Study the drawing (mm; zero at the part's minimum x, y, z) and answer. A direction names the side the tool comes from. Give positions to 0.01 mm unless a question says otherwise; leave off trailing zeros. Order: outer loops, then holes, each group sorted by start corner. A loop starts at its lowest first (then second) coordinate and runs counter-clockwise, first axis right, second up. Notation, with made-up numbers: (-2, 70.25) - (38, 70.25) arc R13 ccw to (38, 88.25) - close; hole circle Ø2 at (49.25, 86). An arc over 180 degrees is marked (long way). Put each result on its own line as item: value.
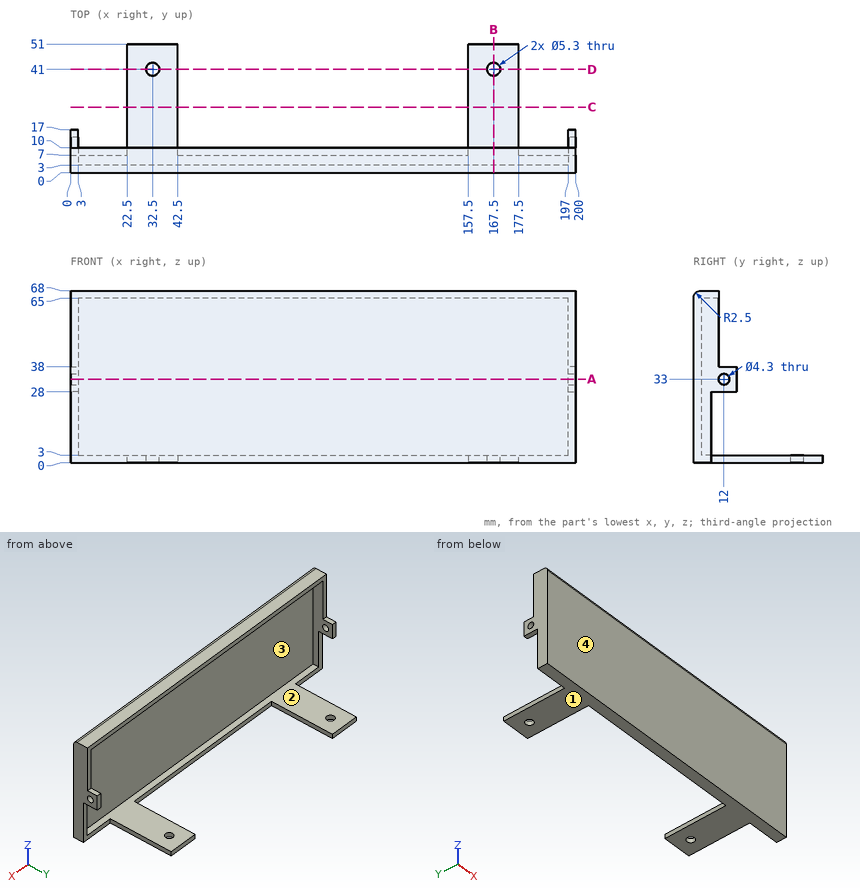
(1) Given pin 1 (18 mm diameter, centred on x = 193, z = 12, fed in from +Y); pin 2 (2.5 mm diameter, centred on y = 19, z = 1.5, fed in from +X); pin 3 (0.9 mm diameter, centred on x = 1, y = 13.5, fed in from -Z); pin 4 (2.5 mm diameter, centred on y = 12, z = 33, fed in from +X), each flat-ended and moving along its own axis, determine where each tip first touches the part or whether it passes through.
Geometry check:
pin 1: stops at y = 7
pin 2: stops at x = 177.5
pin 3: stops at z = 28
pin 4: passes through
(2) Section A-A, the plane z = 33 is taken. Write down the section's boundary in (x, y).
Geometry check:
outline: (0, 0) - (200, 0) - (200, 9.85) - (197, 9.85) - (197, 3) - (3, 3) - (3, 9.85) - (0, 9.85) - close; (0, 14.15) - (3, 14.15) - (3, 17) - (0, 17) - close; (197, 14.15) - (200, 14.15) - (200, 17) - (197, 17) - close
(3) A tool of negligible diameter and unlimited length cuts with its end or side. For the marked faces 3 and 4, from which of +Z, -Z, +X, -X, +Y, -Y can it reach the whole face along a straight path? Write none if from no direction.
Geometry check:
face 3: +Y
face 4: +Z, -Z, +X, -X, -Y
(4) Determine the mould class of the marked faces 1 and 2 for opening direction X: pulls with the +X half, pulls with the -X half, needs draft (parallel to the pull), parting line crosses it, or undercut.
Geometry check:
face 1: needs draft
face 2: undercut
(5) Section C-C, the plane y = 26 is taken. Write down the section's boundary in (x, z).
Geometry check:
outline: (22.5, 0) - (42.5, 0) - (42.5, 3) - (22.5, 3) - close; (157.5, 0) - (177.5, 0) - (177.5, 3) - (157.5, 3) - close
(6) Straight lines are drawn through the part: line 1 (X direction, y = 41, z = 1); line 2 (X direction, y = 9, z = 51); line 3 (Z direction, x = 198, y = 12). For each, find the intervals that lie inside material, in ascending order.
Geometry check:
line 1: x = 22.5 to 29.85, 35.15 to 42.5, 157.5 to 164.85, 170.15 to 177.5
line 2: x = 0 to 3, 197 to 200
line 3: z = 28 to 30.85, 35.15 to 38
(7) Section B-B, the plane x = 167.5 is taken. Write down the section's boundary in (y, z), then the cut area to 3 significant figures.
Geometry check:
outline: (0, 0) - (38.35, 0) - (38.35, 3) - (3, 3) - (3, 65) - (10, 65) - (10, 68) - (2.5, 68) arc R2.5 ccw to (0, 65.5) - close; (43.65, 0) - (51, 0) - (51, 3) - (43.65, 3) - close
area: 352 mm²
(8) Section D-D, the plane y = 41 is taken. Write down the section's boundary in (x, z).
Geometry check:
outline: (22.5, 0) - (29.85, 0) - (29.85, 3) - (22.5, 3) - close; (35.15, 0) - (42.5, 0) - (42.5, 3) - (35.15, 3) - close; (157.5, 0) - (164.85, 0) - (164.85, 3) - (157.5, 3) - close; (170.15, 0) - (177.5, 0) - (177.5, 3) - (170.15, 3) - close
